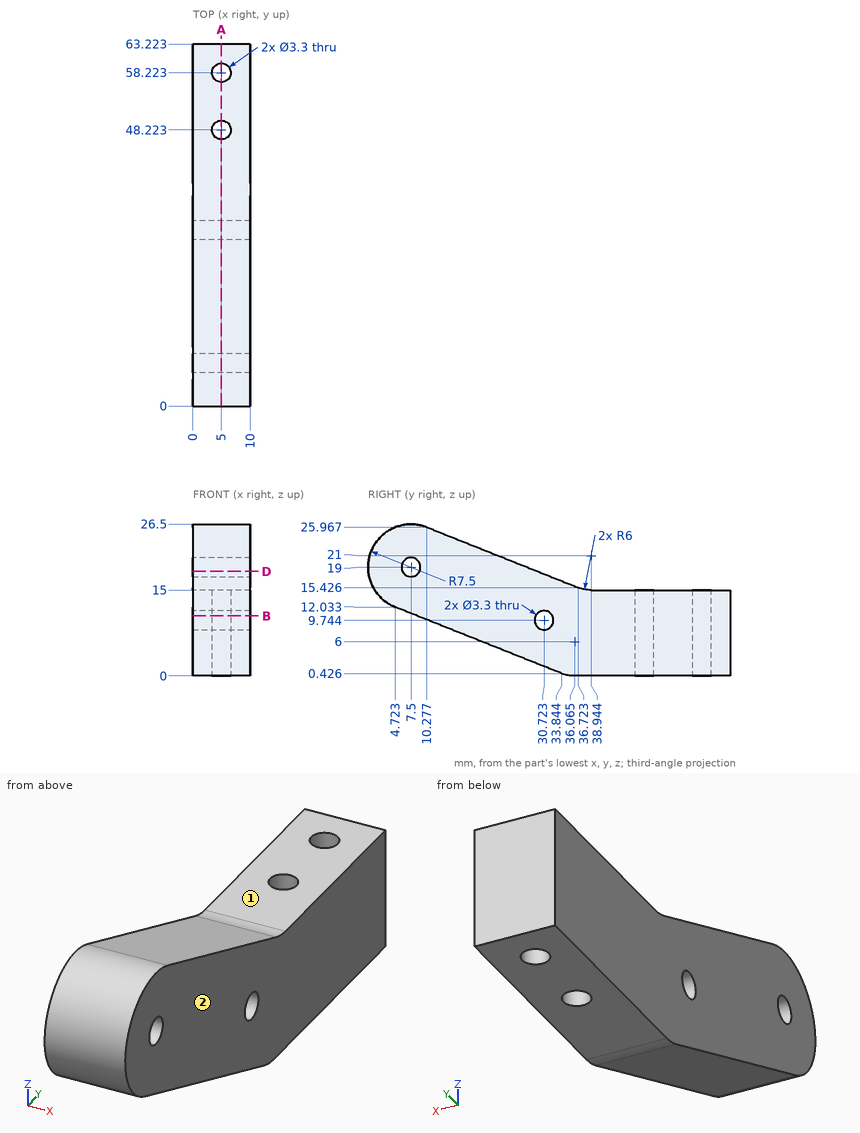
The drawing under review shows one solid part. Ordinate dimensions are in mm from its lowest x, y, z. A direction names the side the tool comes from. Give positions to 0.01 mm unless a question says otherwise; leave off trailing zeros. Order: outer loops, then holes, each group sorted by start corner. A loop starts at its lowest first (then second) coordinate and runs counter-clockwise, first axis right, second up. Notation, with made-up numbers: (38, 63.5) -> (91, 63.5) arc R22 cw to (91, 94.5) -> close; hole circle Ø6 at (-1, 72.5). An arc over 180 degrees is marked (long way). Write item = value, one per line. Start each with the question number.
(1) We need section A-A on x = 5. State how many separate pieces and enclosed holes the cut face has, plus the area to 3 significant figures.
(2) For the marked faces 1 and 2, list the 3-axis set-ups (+Z, -Z, +X, -X, +Y, -Y) from which the entire face can be reached by the end or side of a thin tool; tool diameter is ignored.
(3) We need section B-B on z = 10.5. Write out the cut boundary in (x, y).
(4) For pin 1 (2 mm diameter, centred on x = 5.5, y = 33, fed in from +Z); pin 2 (4 mm diameter, centred on x = 2, y = 38, fed in from +Z) (1 decimal), all flat-tipped, find the tip position at first contact; note any pin that passes through.
(5) We need section D-D on z = 18.25. Write out the cut boundary in (x, y), plus the area to 3 significant figures.
(6) To check wall thickness, follow line 1 along Z through (x, y) = (2.25, 57.5); line 2 along Z through (x, y) = (1.25, 31.5); line 3 along X through (y, z) = (58.5, 6.25). State the ranges of each line that lie inside material, in increasing order.
Numbers:
q1.separate_pieces = 3
q1.enclosed_holes = 2
q1.area = 841 mm^2
q2.face_1 = +Z, +X, -X, +Y
q2.face_2 = +Z, -Z, +X, +Y, -Y
q3.outline = (0, 8.57) -> (10, 8.57) -> (10, 29.26) -> (0, 29.26) -> close; (0, 32.19) -> (10, 32.19) -> (10, 63.22) -> (0, 63.22) -> close; hole circle Ø3.3 at (5, 48.22); hole circle Ø3.3 at (5, 58.22)
q4.pin_1 = 17.31
q4.pin_2 = 15.7
q5.outline = (0, 0.04) -> (10, 0.04) -> (10, 6.03) -> (0, 6.03) -> close; (0, 8.97) -> (10, 8.97) -> (10, 29.64) -> (0, 29.64) -> close
q5.area = 267 mm^2
q6.line_1 = 0 to 15
q6.line_2 = 1.36 to 8.29, 11.2 to 17.51
q6.line_3 = 0 to 3.37, 6.63 to 10
